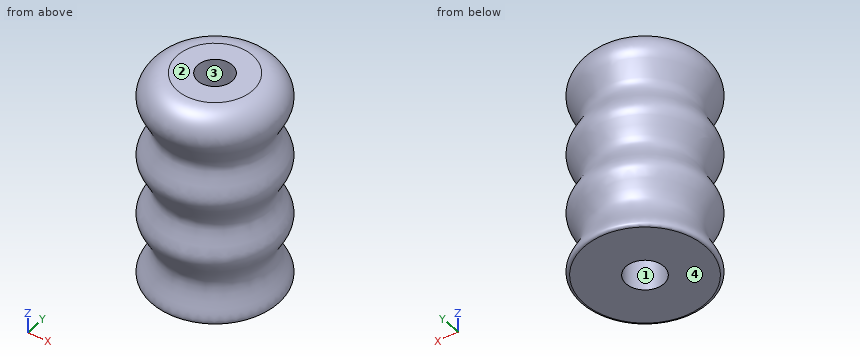
```python
from build123d import *

# Parameters (mm, degrees)
F2_R     = 5.95
F3_DEPTH = 73.0010001
F4_R     = 6.5
F5_DEPTH = 46


with BuildPart() as f1:
    # F0 (on Right) → F1 (revolve)
    with BuildSketch(Plane.YZ):
        with BuildLine():
            Line((0, 73), (0, 0))
            Line((0, 0), (21, 0))
            add(Edge.make_bspline(
                [(13, 73), (18.136955159, 73), (25.9599337866, 64.0409360544), (14.06615934, 54.0451662341), (25.9802216397, 43.3505110298), (14.0129541012, 32.9527896469), (25.9679619557, 22.2383303828), (14.1151980762, 12.4938888218), (23.2468316742, 1.8862408584), (21.646819451, 0), (21, 0)],
                knots=[0, 0, 0, 0, 0.1413997222, 0.2757385334, 0.4100773447, 0.544416156, 0.6787549672, 0.8130937785, 0.9474325897, 1, 1, 1, 1], degree=3))
            Line((13, 73), (0, 73))
        make_face()
    revolve(axis=Axis((0, 0, 36.5), (0, 0, 1)))

    # F2 (on face) → F3 (cut, through all)
    with BuildSketch(Plane.XY.offset(73)):
        Circle(F2_R)
    extrude(amount=-F3_DEPTH, mode=Mode.SUBTRACT)

    # F4 (on face) → F5 (cut)
    with BuildSketch(Plane(origin=(0, 0, 0), x_dir=(1, 0, 0), z_dir=(0, 0, -1))):
        Circle(F4_R)
    extrude(amount=-F5_DEPTH, mode=Mode.SUBTRACT)


solid = f1.part
```
Can you work these out from the model? Positions are in its coordinate system, mm. Face numbers are marked on the shaded views. A direction names the side the tool comes from. Give positions to 0.01 mm unless a question says otherwise; leave off trailing zeros. Answer in a Markdown table with one row per item.
1. Which directions (+Z, -Z, +X, -X, +Y, -Y) give clear straight access to the entire face, cutting with the end or side of a thin tool? Please do the marked faces 1 and 2.
Taken from the geometry:
| item | result |
|---|---|
| face 1 | -Z |
| face 2 | +Z, +X, -X, +Y, -Y |
2. Suppose I cut it at A-A on x = -18.5. Count the separate pieces of the cut face and the enclosed holes in it, plus the area to 3 significant figures.
Taken from the geometry:
| item | result |
|---|---|
| separate pieces | 4 |
| enclosed holes | 0 |
| area | 966 mm² |
3. Thinking about a two-plate mould opening in Y: for the marked faces 3 and 4, which applies, released by +Y, released by -Y, zero draft, split by the parting line, or undercut?
Taken from the geometry:
| item | result |
|---|---|
| face 3 | undercut |
| face 4 | zero draft |
4. For pin 1 Ø10 at (x, z) = (3, 48.5) entering from -Y; pin 2 Ø1 at (y, z) = (12.5, 21.5) entering from +X; pin 3 Ø4 at (x, z) = (16, 20) entering from +Y, each with a flat end and sliding along its axis, tell me the tip position at first contact or that it passes through.
Taken from the geometry:
| item | result |
|---|---|
| pin 1 | stops at y = -21.95 |
| pin 2 | stops at x = 18.36 |
| pin 3 | stops at y = 16.5 |
5. If I drill on line 1 along Z through (x, y) = (-13, -15); line 2 along Z through (x, y) = (18, -8); line 3 along X through (y, z) = (-1, 7), over which ranges is the centre line in solid material (lowest first)?
Taken from the geometry:
| item | result |
|---|---|
| line 1 | z = 0 to 6.11, 17 to 27.86, 37.89 to 48.98, 58.86 to 69.81 |
| line 2 | z = 0 to 6.4, 16.73 to 28.13, 37.63 to 49.25, 58.59 to 69.98 |
| line 3 | x = -19.37 to -6.42, 6.42 to 19.37 |
